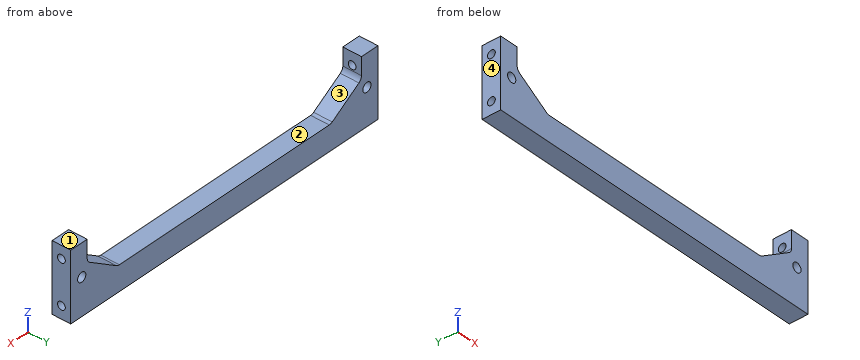
```python
from build123d import *

# Parameters (mm, degrees)
SKETCH1_R                        = 1.5
BOSS_EXTRUDE1_DEPTH              = 6
FILLET1_R                        = 2
TAP_DRILL_FOR_M3_TAP1_AT_2_COUNT = 2
TAP_DRILL_FOR_M3_TAP1_AT_2_PITCH = 14
FILLET1_OF_MIRROR1_R             = 2


with BuildPart() as part:
    # Sketch1 → Boss-Extrude1 (new body)
    with BuildSketch(Plane(origin=(0, 0, 0), x_dir=(1, 0, 0), z_dir=(0, 1, 0))):
        Polygon((0, -22), (-56, -22), (-56, -44), (-50, -44), (-50, -37.239832831), (-38.851635079, -30), (0, -30), align=None)
        with Locations(Location((-51.997575213, -33.767620171, 0), (0, 0, 270))):
            Circle(SKETCH1_R, mode=Mode.SUBTRACT)
    boss_extrude1 = extrude(amount=BOSS_EXTRUDE1_DEPTH)

    # Fillet1
    fillet1_edges = [part.edges().sort_by_distance(p)[0] for p in [
        (-38.851635079, 3, 30),
        (-50, 3, 37.239832831),
    ]]
    fillet(fillet1_edges, radius=FILLET1_R)

    # Sketch2 → Tap Drill for M3 Tap1 (revolve, cut)
    with BuildSketch(Plane(origin=(-56, 3, 26), x_dir=(0, 0, 1), z_dir=(0, 1, 0))):
        Polygon((0, 0), (0, 10.751075774), (1.25, 10), (1.25, 0), align=None)
    tap_drill_for_m3_tap1 = revolve(axis=Axis((-62.35, 3, 26), (1, 0, 0)), mode=Mode.SUBTRACT)

    # Tap Drill for M3 Tap1 at 2: Tap Drill for M3 Tap1 ×2
    with Locations(*[(0, 0, i * TAP_DRILL_FOR_M3_TAP1_AT_2_PITCH) for i in range(1, TAP_DRILL_FOR_M3_TAP1_AT_2_COUNT)]):
        add(tap_drill_for_m3_tap1, mode=Mode.SUBTRACT)

    # Mirror1: Boss-Extrude1, Tap Drill for M3 Tap1 across plane
    add(boss_extrude1.mirror(Plane(origin=(0, 6, 30), x_dir=(0, 0, 1), z_dir=(-1, 0, 0))))
    add(tap_drill_for_m3_tap1.mirror(Plane(origin=(0, 6, 30), x_dir=(0, 0, 1), z_dir=(-1, 0, 0))), mode=Mode.SUBTRACT)

    # Mirror1 copy 1 sketch → Mirror1 copy 1 (revolve, cut)
    with BuildSketch(Plane(origin=(56, 3, 40), x_dir=(0, 0, 1), z_dir=(0, 1, 0))):
        Polygon((0, 0), (0, -10.751075774), (1.25, -10), (1.25, 0), align=None)
    revolve(axis=Axis((62.35, 3, 40), (1, 0, 0)), mode=Mode.SUBTRACT)

    # Fillet1 of Mirror1
    fillet1_of_mirror1_edges = [part.edges().sort_by_distance(p)[0] for p in [
        (38.851635079, 3, 30),
        (50, 3, 37.239832831),
    ]]
    fillet(fillet1_of_mirror1_edges, radius=FILLET1_OF_MIRROR1_R)


solid = part.part
```
Input: part model. Units: mm. Frame: model coordinates. Face numbers are marked on the shaded views. Give positions to 0.01 mm unless a question says otherwise; leave off trailing zeros. Order: outer loops, then holes, each group sorted by start corner. A loop starts at its lowest first (then second) coordinate and runs counter-clockwise, first axis right, second up. Notation, with made-up numbers: (61, 53.5) - (95, 53.5) arc R21 cw to (95, 60.5) - close; hole circle Ø2 at (45.5, 10). An arc over 180 degrees is marked (long way). Use a Markdown table: item, result.
(1) Pin query (flat end, axial travel): pin 1 (1 mm diameter, centred on x = -35.5, y = 3.5, fed in from +Z); pin 2 (3.5 mm diameter, centred on x = 52, z = 33.77, fed in from +Y); pin 3 (2.5 mm diameter, centred on x = -52, z = 33.77, fed in from -Y); pin 4 (1 mm diameter, centred on x = -38.5, y = 3, fed in from +Z). Return the tip coordinate at first contact, or that it passes through.
Computed values:
| item | result |
|---|---|
| pin 1 | stops at z = 30 |
| pin 2 | stops at y = 6 |
| pin 3 | passes through |
| pin 4 | stops at z = 30.14 |
(2) Section query A-A (z = 40). Output: boundary loops of the cut face in (x, y), then the cut area to 3 significant figures.
Computed values:
| item | result |
|---|---|
| outline | (-56, 0) - (-50, 0) - (-50, 1.75) - (-56, 1.75) - close; (-56, 4.25) - (-50, 4.25) - (-50, 6) - (-56, 6) - close; (50, 0) - (56, 0) - (56, 1.75) - (50, 1.75) - close; (50, 4.25) - (56, 4.25) - (56, 6) - (50, 6) - close |
| area | 42.0 mm2 |
(3) Section query B-B (x = 30). Output: boundary loops of the cut face in (y, z).
Computed values:
| item | result |
|---|---|
| outline | (0, 22) - (6, 22) - (6, 30) - (0, 30) - close |
(4) Section query C-C (x = -41). Output: boundary loops of the cut face in (y, z), then the cut area to 3 significant figures.
Computed values:
| item | result |
|---|---|
| outline | (0, 22) - (6, 22) - (6, 31.4) - (0, 31.4) - close |
| area | 56.4 mm2 |
(5) Draft query along X for the marked faces 1, 2, 3 and 4. Return one class per face: released by +X, released by -X, zero draft, split by the parting line, or undercut.
Computed values:
| item | result |
|---|---|
| face 1 | zero draft |
| face 2 | undercut |
| face 3 | undercut |
| face 4 | released by -X |
(6) Line query: line 1 (Z direction, x = 52.25, y = 3); line 2 (X direction, y = 3.75, z = 41.5); line 3 (X direction, y = 2.05, z = 34.5). Output: solid intervals per line, ascending. Write a range as from..to.
Computed values:
| item | result |
|---|---|
| line 1 | z = 22..24.75, 27.25..32.29, 35.25..38.75, 41.25..44 |
| line 2 | x = -56..-50, 50..56 |
| line 3 | x = -56..-53.31, -50.69..-45.78, 45.78..50.69, 53.31..56 |
